For this review, use the dimensioned drawing (mm, ordinates from the lowest corner) and the shaded views. A direction names the side the tool comes from. Round coordinates to 2 decimals unless told otherwise and drop trailing zeros. Order: outer loops, then holes, each group sorted by start corner. A loop starts at its lowest first (then second) coordinate and runs counter-clockwise, first axis right, second up. Notation, with made-up numbers: (55, 58.5) -> (98, 58.5) arc R19 cw to (98, 84.5) -> close; hole circle Ø11 at (23.5, -10). An arc over 180 degrees is marked (long way). Use a Markdown table: item, result. Add a question column.
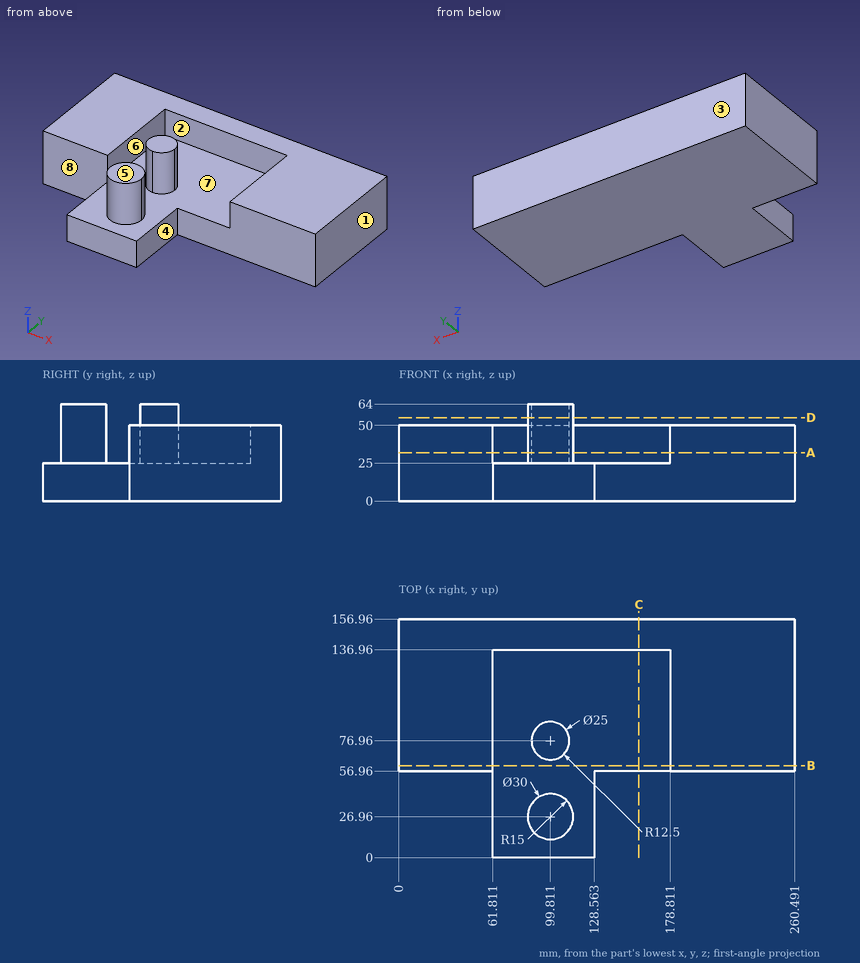
Q1. Add section A-A (z = 32). Write out the cut boundary in (x, y), then the cut area to 3 significant figures.
Q2. Add section B-B (y = 60.5). Write out the cut boundary in (x, z).
Q3. Machinability: for the marked faces 4, 5, 6, 7 and 8, which of the approach directions +Z, -Z, +X, -X, +Y, -Y give a long, thin tool a straight path to every point of the face, cutting with its end or side? Answer none if there is none.
Q4. Add section C-C (x = 158). Write out the cut boundary in (y, z).
Q5. Wall thickness on line 1 (X direction, y = 133, z = 42.5); line 2 (X direction, y = 74.5, z = 32) (1 decimal); line 3 (Y direction, x = 13.5, z = 42.5): over which ranges is each line inside the solid? List them lowest first. Write a range as [from, to].
Q6. Insertion check: pin 1 (1 mm diameter, centred on x = 83, y = 107.5, fed in from +Z); pin 2 (20 mm diameter, centred on x = 107.5, z = 39, fed in from -Y); pin 3 (7.5 mm diameter, centred on y = 41, z = 10.5, fed in from +X). Each pin has a flat end and moves straight along its axis. Give the tip position at first contact, or say it passes through.
Q7. Add section D-D (z = 55). Write out the cut boundary in (x, y), then the cut area to 3 significant figures.
Q8. Mouldability with a two-part tool opening along Y and no side actions: class the marked faces 1, 2 and 3 as pulls with the +Y half, pulls with the -Y half, needs draft (parallel to the pull), parting line crosses it, or undercut.
Report:
| question | item | result |
|---|---|---|
| 1 | outline | (0, 56.96) -> (61.81, 56.96) -> (61.81, 136.96) -> (178.81, 136.96) -> (178.81, 56.96) -> (260.49, 56.96) -> (260.49, 156.96) -> (0, 156.96) -> close; circle Ø30 at (99.81, 26.96); circle Ø25 at (99.81, 76.96) |
| 1 | area | 17,900 mm² |
| 2 | outline | (0, 0) -> (260.49, 0) -> (260.49, 50) -> (178.81, 50) -> (178.81, 25) -> (61.81, 25) -> (61.81, 50) -> (0, 50) -> close |
| 3 | face 4 | +Z, -Z, +X, -Y |
| 3 | face 5 | +Z, +X, -X, +Y, -Y |
| 3 | face 6 | +Z, -Y |
| 3 | face 7 | +Z |
| 3 | face 8 | +Z, -Z, -X, -Y |
| 4 | outline | (56.96, 0) -> (156.96, 0) -> (156.96, 50) -> (136.96, 50) -> (136.96, 25) -> (56.96, 25) -> close |
| 5 | line 1 | x = [0, 61.81], [178.81, 260.49] |
| 5 | line 2 | x = [0, 61.8], [87.6, 112.1], [178.8, 260.5] |
| 5 | line 3 | y = [56.96, 156.96] |
| 6 | pin 1 | stops at z = 25 |
| 6 | pin 2 | stops at y = 11.96 |
| 6 | pin 3 | stops at x = 128.56 |
| 7 | outline | circle Ø30 at (99.81, 26.96); circle Ø25 at (99.81, 76.96) |
| 7 | area | 1,200 mm² |
| 8 | face 1 | needs draft |
| 8 | face 2 | undercut |
| 8 | face 3 | pulls with the +Y half |
